Work out the finished part from the listing and answer in its coordinate system (mm). Round coordinates to 2 decimals unless told otherwise and drop trailing zeros. Order: outer loops, then holes, each group sorted by start corner. A loop starts at its lowest first (then second) coordinate and runs counter-clockwise, first axis right, second up. Notation, with made-up numbers: (-34.75, 5) - (-14.75, 5) arc R12 ccw to (-14.75, 10) - close; hole circle Ø8 at (13.25, -36.5). An arc over 180 degrees is marked (long way). Use CSV: the item, a comma, the result in double quotes.
from build123d import *

# Parameters (mm, degrees)
F0_W     = 150
F0_H     = 140
F1_DEPTH = 86
F3_DEPTH = 25


with BuildPart() as f1:
    # F0 (on Top) → F1 (new body)
    with BuildSketch(Plane.XY):
        Rectangle(F0_W, F0_H)
    extrude(amount=F1_DEPTH)

    # F2 (on face) → F3 (cut)
    with BuildSketch(Plane.XZ.offset(70)):
        with BuildLine():
            ThreePointArc((50, 61), (39.393398, 35.393398), (65, 46))
            Line((65, 46), (50, 46))
            Line((50, 46), (50, 61))
        make_face()
        with BuildLine():
            Line((50, 46), (65, 46))
            ThreePointArc((65, 46), (60.606602, 56.606602), (50, 61))
            Line((50, 61), (50, 46))
        make_face()
    extrude(amount=-F3_DEPTH, mode=Mode.SUBTRACT)


solid = f1.part
(1) This flat-tipped pin is pushed along its axis until it touches: pin 1 (3 mm diameter, centred on x = -31, y = -46, fed in from -Z). Where does it stop, or does it pass through?
Findings below:
pin 1,"stops at z = 0"
(2) Find section C-C (x = 60.5). Determine the outline of the cut face in (y, z).
Findings below:
outline,"(-70, 0) - (70, 0) - (70, 86) - (-70, 86) - (-70, 56.71) - (-45, 56.71) - (-45, 35.29) - (-70, 35.29) - close"
(3) The mould has two halves that part along X. Classify faces 1 (the flat face through (-75, -1, 42)), 2 (the flat face through (75, -1, 42)), 3 (the flat face through (50, -45, 46)), 4 (the flat face through (-1, 70, 42)): released by +X, released by -X, zero draft, split by the parting line, or undercut.
Findings below:
face 1,"released by -X"
face 2,"released by +X"
face 3,"undercut"
face 4,"zero draft"
(4) Find section B-B (z = 54). Determine the outline of the cut face in (x, y).
Findings below:
outline,"(-75, -70) - (37.31, -70) - (37.31, -45) - (62.69, -45) - (62.69, -70) - (75, -70) - (75, 70) - (-75, 70) - close"
(5) Find section A-A (y = -50). Determine the outline of the cut face in (x, z), and give its area (3 significant figures).
Findings below:
outline,"(-75, 0) - (75, 0) - (75, 86) - (-75, 86) - close; hole (50, 61) arc R15 ccw (long way) to (65, 46) arc R15 ccw to start"
area,"12,200 mm²"
(6) Find the intervals of material crossed by L1, parallel to Z at x = 50, y = -65; L2, parallel to X at y = -53, z = 46, in increasing order. Write a range as from..to.
Findings below:
L1,"z = 0..31, 61..86"
L2,"x = -75..35, 65..75"
